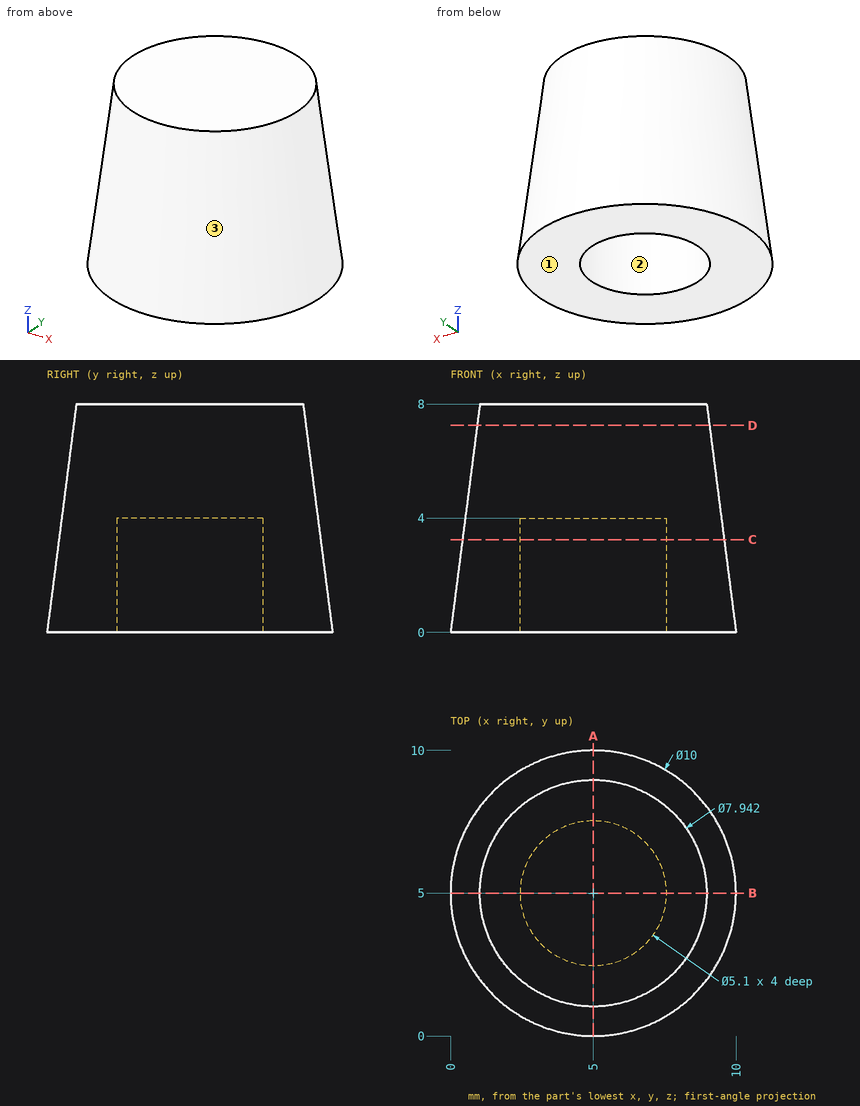
Source: three-view drawing plus pictorial views. Frame: mm from the lowest corner of the part. Give positions to 0.01 mm unless a question says otherwise; leave off trailing zeros. Order: outer loops, then holes, each group sorted by start corner. A loop starts at its lowest first (then second) coordinate and runs counter-clockwise, first axis right, second up. Notation, with made-up numbers: M 79,42 L 108,42 A5 ccw 108,46 Z; hole C 50,26.25 d3. An arc over 180 degrees is marked long. One line per question, with ' | ' between items. Start each with the question number.
1. Section query D-D (z = 7.25). Return the cut outline in (x, y) (1 decimal), and give its area (3 significant figures).
2. Material intervals for probe 1 along Z at (x, y) = (6.75, 3.75); probe 2 along Y at (x, z) = (5, 3); probe 3 along Y at (x, z) = (5, 2.45) (3 decimals), sorted ascending. Write a range as [from, to].
3. Section query C-C (z = 3.25). Return the cut outline in (x, y), and give its area (3 significant figures).
4. Pull-direction query (Y, two-part tool) for the marked faces 1, 2 and 3; classes: released by +Y, released by -Y, zero draft, split by the parting line, or undercut.
5. Section query A-A (x = 5). Return the cut outline in (y, z), and give its area (3 significant figures).
6. First-contact query: pin 1 Ø3 at (y, z) = (2.5, 5.5) entering from +X; pin 2 Ø4 at (x, z) = (6.5, 2.5) entering from +Y; pin 3 Ø1 at (x, z) = (5.5, 4.5) entering from +Y. Flat tips, straight axial feed; report the tip coordinate or a pass-through.
Here are the results:
1) outline: C 5,5 d8.1 | area: 52.0 mm²
2) probe 1: [4, 8] | probe 2: [0.39, 2.45], [7.55, 9.61] | probe 3: [0.315, 2.45], [7.55, 9.685]
3) outline: C 5,5 d9.16; hole C 5,5 d5.1 | area: 45.5 mm²
4) face 1: zero draft | face 2: undercut | face 3: split by the parting line
5) outline: M 0,0 L 2.45,0 L 2.45,4 L 7.55,4 L 7.55,0 L 10,0 L 8.97,8 L 1.03,8 Z | area: 51.4 mm²
6) pin 1: x = 9.22 | pin 2: y = 9.88 | pin 3: y = 9.47
